```python
from build123d import *

# Parameters (mm, degrees)
F0_W     = 50
F0_H     = 20
F0_W_2   = 46
F0_H_2   = 16
F1_DEPTH = 550
F2_R     = 3
F3_DEPTH = 50.001
F5_DEPTH = 20.001


# Not quite as in the source:
# - a pattern or mirror of a feature is missing from the dataset's text; its kind, count and spacing are read off the source's solid


with BuildPart() as f1:
    # F0 (on Right) → F1 (new body)
    with BuildSketch(Plane.YZ):
        with Locations((25, 10)):
            Rectangle(F0_W, F0_H)
        with Locations((25, 10)):
            Rectangle(F0_W_2, F0_H_2, mode=Mode.SUBTRACT)
    extrude(amount=F1_DEPTH)

    # F2 (on face) → F3 (cut, through all)
    with BuildSketch(Plane.XZ):
        with Locations((10, 10)):
            Circle(F2_R)
        with Locations((540, 10)):
            Circle(F2_R)
    extrude(amount=-F3_DEPTH, mode=Mode.SUBTRACT)

    # F4 (on face) → F5 (cut, through all)
    with BuildSketch(Plane.XY.offset(20)):
        with BuildLine():
            Line((0, 11.5), (49, 11.5))
            ThreePointArc((49, 11.5), (62.5, 25), (49, 38.5))
            Line((49, 38.5), (0, 38.5))
            Line((0, 38.5), (0, 11.5))
        make_face()
    f5 = extrude(amount=-F5_DEPTH, mode=Mode.SUBTRACT)

    # F5_copies: F5 across plane
    add(f5.mirror(Plane(origin=(275, 0, 0), x_dir=(0, 0, 1), z_dir=(1, 0, 0))), mode=Mode.SUBTRACT)


solid = f1.part
```
Model file for the job. Use its own axes, mm. A direction names the side the tool comes from. Coordinates: 2 decimals unless noted, no trailing zeros. Order: outer loops, then holes, each group sorted by start corner. A loop starts at its lowest first (then second) coordinate and runs counter-clockwise, first axis right, second up. Notation, with made-up numbers: (-1, 1) -> (25, 1) arc R23 ccw to (25, 23) -> close; hole circle Ø1 at (-33.5, -29). An arc over 180 degrees is marked (long way). Return JSON: item names as keys, results as strings.
Item 1: Slice it at B-B (x = 182). Write the cut outline in (y, z).
Model answer:
{"outline": "(0, 0) -> (50, 0) -> (50, 20) -> (0, 20) -> close; hole (2, 2) -> (48, 2) -> (48, 18) -> (2, 18) -> close"}
Item 2: Slice it at A-A (y = 43). Write the cut outline in (x, z).
Model answer:
{"outline": "(0, 0) -> (550, 0) -> (550, 2) -> (0, 2) -> close; (0, 18) -> (550, 18) -> (550, 20) -> (0, 20) -> close"}
Item 3: Pin check, flat tips, straight feed: P1, Ø2, axis at x = 13.5, z = 0.5, coming from the -Y side; P2, Ø3.5, axis at x = 540, z = 10, coming from the -Y side; P3, Ø10, axis at y = 26.5, z = 6.5, coming from the -X side. Stop position of each tip, or through.
Model answer:
{"P1": "stops at y = 0", "P2": "passes through", "P3": "stops at x = 61.99"}
Item 4: Slice it at C-C (y = 18). Write the cut outline in (x, z), then the cut area to 3 significant figures.
Model answer:
{"outline": "(60.54, 0) -> (489.46, 0) -> (489.46, 2) -> (60.54, 2) -> close; (60.54, 18) -> (489.46, 18) -> (489.46, 20) -> (60.54, 20) -> close", "area": "1,720 mm²"}
Item 5: Mould opens along Y. For faces 3 (the face through (271, 25, 20)), 4 (the face through (487.503, 24.703, 19.014)), 5 (the face through (271, 0, 10)) say: pulls with the +Y half, pulls with the -Y half, needs draft (parallel to the pull), parting line crosses it, or undercut.
Model answer:
{"face 3": "needs draft", "face 4": "undercut", "face 5": "pulls with the -Y half"}
Item 6: 3-axis set-ups, long thin cutter, end or side, ignore diameter. For faces 1 (the face through (0, 49, 10)), 2 (the face through (271, 48, 10)): which of +Z, -Z, +X, -X, +Y, -Y reach the whole face in a straight line?
Model answer:
{"face 1": "+Z, -Z, -X, +Y, -Y", "face 2": "+X, -X"}
Item 7: Wall check: line 1 along Z through (x, y) = (10, 48.5); line 2 along Y through (x, z) = (346.5, 17.5); line 3 along Z through (x, y) = (311, 35). Give the ranges that are in metal, low to high. Write a range as from..to.
Model answer:
{"line 1": "z = 0..7, 13..20", "line 2": "y = 0..2, 48..50", "line 3": "z = 0..2, 18..20"}
